Could you check a few things on this model? Use its own coordinates, in mm. A direction names the side the tool comes from. Coordinates: 2 decimals unless noted, no trailing zeros. Order: outer loops, then holes, each group sorted by start corner. A loop starts at its lowest first (then second) coordinate and runs counter-clockwise, first axis right, second up. Notation, with made-up numbers: M 16,76.25 L 66,76.25 A15 ccw 66,84.25 Z; hole C -2,-30 d9. An arc over 180 degrees is marked long. One line per question, with ' | ' between items. Start each with the question number.
from build123d import *

# Parameters (mm, degrees)
SKETCH1_W           = 45.72
SKETCH1_H           = 58.42
BOSS_EXTRUDE1_DEPTH = 12.7
SKETCH2_R           = 1.905
CUT_EXTRUDE1_DEPTH  = 42.348948188
SKETCH3_W           = 36.327462092
SKETCH3_H           = 46.418423785
BOSS_EXTRUDE2_DEPTH = 5.08
SKETCH4_R           = 7.62
SKETCH4_R_2         = 5.08
BOSS_EXTRUDE3_DEPTH = 12.7
FILLET1_R           = 2.54


with BuildPart() as part:
    # Sketch1 → Boss-Extrude1 (new body)
    with BuildSketch(Plane(origin=(0, 0, 0), x_dir=(1, 0, 0), z_dir=(0, 1, 0))):
        with Locations((2.874210526, -0.559043062)):
            Rectangle(SKETCH1_W, SKETCH1_H)
    extrude(amount=BOSS_EXTRUDE1_DEPTH)

    # Sketch2 → Cut-Extrude1 (cut, through all)
    with BuildSketch(Plane(origin=(0, 12.7, 0), x_dir=(1, 0, 0), z_dir=(0, 1, 0))):
        with Locations(Location((-8.555789474, 14.045956938, 0), (0, 0, 270))):
            Circle(SKETCH2_R)
        with Locations(Location((14.304210526, 14.045956938, 0), (0, 0, 270))):
            Circle(SKETCH2_R)
        with Locations(Location((-8.555789474, -15.164043062, 0), (0, 0, 270))):
            Circle(SKETCH2_R)
        with Locations(Location((14.304210526, -15.164043062, 0), (0, 0, 270))):
            Circle(SKETCH2_R)
    extrude(amount=-CUT_EXTRUDE1_DEPTH, mode=Mode.SUBTRACT)

    # Sketch3 → Boss-Extrude2 (add)
    with BuildSketch(Plane.XZ):
        with Locations((2.874210526, 0.559043062)):
            Rectangle(SKETCH3_W, SKETCH3_H)
    extrude(amount=BOSS_EXTRUDE2_DEPTH)

    # Sketch4 → Boss-Extrude3 (add)
    with BuildSketch(Plane.XZ.offset(5.08)):
        with Locations(Location((2.874210526, 0.559043062, 0), (0, 0, 270))):
            Circle(SKETCH4_R)
        with Locations(Location((2.874210526, 0.559043062, 0), (0, 0, 270))):
            Circle(SKETCH4_R_2, mode=Mode.SUBTRACT)
    extrude(amount=BOSS_EXTRUDE3_DEPTH)

    # Fillet1
    fillet1_edges = [part.edges().sort_by_distance(p)[0] for p in [
        (-19.985789474, 6.35, -28.650956938),
        (25.734210526, 6.35, -28.650956938),
        (25.734210526, 6.35, 29.769043062),
        (-19.985789474, 6.35, 29.769043062),
    ]]
    fillet(fillet1_edges, radius=FILLET1_R)


solid = part.part
(1) On a 3-axis mill with a long thin cutter (end or side, diameter ignored), from which of +Z, -Z, +X, -X, +Y, -Y can I reach the whole of each face in a straight line? I mean faces 1 (the flat face through (3, -3, 23.768)), 2 (the flat face through (-19.986, 6, 1)), 3 (the flat face through (14, 0, 15)), 4 (the flat face through (3, -3, -22.65)), 5 (the flat face through (25.734, 6, 1)). Say none if no direction works.
(2) We'd pull the mould along Z, two halves only. Please class faces 6 (the cylindrical face through (-1.76, -11.34, 6.61)), 7 (the flat face through (3, 12.7, 0)), 8 (the flat face through (14, 0, -14)): +Z half, -Z half, draft (parallel to the pull), parting line (faces both ways), or undercut.
(3) Imagine slicing it at C-C, the plane y = 5. Write out the boundary of the cut face in (x, z) (3 decimals).
(4) For P1, Ø3.5, axis at x = -8.56, z = -14.05, coming from the +Y side; P2, Ø4, axis at y = -3, z = -11, coming from the +X side; P3, Ø8, axis at x = -8.5, z = -4, coming from the -Y side, each with a flat end and sliding along its axis, tell me the tip position at first contact or that it passes through.
(5) Imagine slicing it at A-A, the plane z = -9. Write out the boundary of the cut face in (x, y), plus the area to 3 significant figures.
(6) If I drill on line 1 along Y through (x, z) = (0, -17); line 2 along X through (y, z) = (2.5, -15); line 3 along X through (y, z) = (-4, 17), over which ranges is the centre line in solid material (lowest first)? Write a range as from..to.
(7) Imagine slicing it at D-D, the plane y = -14.5. Write out the boundary of the cut face in (x, z).
(8) Imagine slicing it at B-B, the plane x = -5.5. Write out the boundary of the cut face in (y, z), plus the area to 3 significant figures.
Answers:
1) face 1: +Z, +X, -X, -Y | face 2: +Z, -Z, -X, +Y, -Y | face 3: +Y | face 4: -Z, +X, -X, -Y | face 5: +Z, -Z, +X, +Y, -Y
2) face 6: parting line | face 7: draft | face 8: undercut
3) outline: M -19.986,-26.111 A2.54 ccw -17.446,-28.651 L 23.194,-28.651 A2.54 ccw 25.734,-26.111 L 25.734,27.229 A2.54 ccw 23.194,29.769 L -17.446,29.769 A2.54 ccw -19.986,27.229 Z; hole C -8.556,-14.046 d3.81; hole C -8.556,15.164 d3.81; hole C 14.304,-14.046 d3.81; hole C 14.304,15.164 d3.81
4) P1: y = 0 | P2: x = 21.04 | P3: y = -5.08
5) outline: M -19.99,0 L -15.29,0 L -15.29,-5.08 L 21.04,-5.08 L 21.04,0 L 25.73,0 L 25.73,12.7 L -19.99,12.7 Z | area: 765 mm²
6) line 1: -5.08..12.7 | line 2: -19.99..-10.2, -6.91..12.66, 15.95..25.73 | line 3: -15.29..21.04
7) outline: C 2.87,0.56 d15.24; hole C 2.87,0.56 d10.16
8) outline: M -5.08,-22.65 L 0,-22.65 L 0,-28.65 L 12.7,-28.65 L 12.7,29.77 L 0,29.77 L 0,23.77 L -5.08,23.77 Z | area: 978 mm²
